Work out the finished part from the listing and answer in its coordinate system (mm). A direction names the side the tool comes from. Round coordinates to 2 decimals unless told otherwise and drop trailing zeros. Write each loop counter-clockwise with the first axis right and the second up, starting at its lowest first coordinate (ties: lowest second). Pieces come first, ordered by that corner, then holes.
1. Find section A-A (x = 0). Write down the section's boundary in (y, z).
2. Straight lines are drawn through the part: probe 1 along X at (y, z) = (2, 9); probe 2 along Z at (x, y) = (-33, 10); probe 3 along Y at (x, z) = (-16, 5). For each, find the intervals that lie inside material, in ascending order.
3. Flat-ended cylindrical pins translate along their axes: pin 1 Ø2 at (x, z) = (-28, -16) entering from -Y; pin 2 Ø4 at (x, z) = (-35, 8) entering from +Y; pin 3 Ø4.5 at (x, z) = (-37, 5.5) entering from +Y; pin 4 Ø2.5 at (x, z) = (-15.63, -6.22) entering from +Y. Find the tip coordinate at first contact, or state that the pin passes through.
4. Find section C-C (z = -2). Write down the section's boundary in (x, y).
5. Find section D-D (z = -24). Count the separate pieces of the cut face and the enclosed holes in it, and give its area (3 significant figures).
6. Find section B-B (y = 9.5). Write down the section's boundary in (x, z).
7. A tool of negligible diameter and unlimited length cuts with its end or side. For faces 5 (the face through (35, 5, -7)), 6 (the face through (-34, 3.75, 12)), 7 (the face through (-22.5, 10, -7)), 8 (the face through (-33, 9, 19)), from which of +Z, -Z, +X, -X, +Y, -Y can it reach the whole face along a straight path? Write none if from no direction.
8. Determine the mould class of faces 1 (the face through (-34, 3.75, -21)), 2 (the face through (-35, 5, -7)), 3 (the face through (-42.434, 2, -7)), 4 (the face through (28.36, 15.48, -33.1)) for opening direction X: pulls with the +X half, pulls with the -X half, needs draft (parallel to the pull), parting line crosses it, or undercut.
```python
from build123d import *

# Parameters (mm, degrees)
SKETCH1_W           = 50
SKETCH1_H           = 50
BOSS_EXTRUDE1_DEPTH = 30
SKETCH2_R           = 7
CUT_EXTRUDE1_DEPTH  = 30
SKETCH3_R           = 1.7
CUT_EXTRUDE2_DEPTH  = 42
SKETCH5_W           = 50
SKETCH5_H           = 15
BOSS_EXTRUDE2_DEPTH = 30
BOSS_EXTRUDE3_DEPTH = 65
SKETCH7_W           = 45
SKETCH7_H           = 42.253035939
CUT_EXTRUDE3_DEPTH  = 66
FILLET1_R           = 4
CUT_EXTRUDE4_DEPTH  = 53
SKETCH10_R          = 4
CUT_EXTRUDE5_DEPTH  = 1.25
SKETCH11_R          = 2.5
CUT_EXTRUDE6_DEPTH  = 36.25
CUT_EXTRUDE7_DEPTH  = 90.25
FILLET2_R           = 3
SKETCH13_W          = 3
SKETCH13_H          = 5
BOSS_EXTRUDE4_DEPTH = 65
FILLET3_R           = 3


with BuildPart() as part:
    # Sketch1 → Boss-Extrude1 (new body)
    with BuildSketch(Plane(origin=(0, 0, 0), x_dir=(1, 0, 0), z_dir=(0, 1, 0))):
        Rectangle(SKETCH1_W, SKETCH1_H)
    extrude(amount=BOSS_EXTRUDE1_DEPTH)

    # Sketch2 → Cut-Extrude1 (cut)
    with BuildSketch(Plane(origin=(0, 30, 0), x_dir=(1, 0, 0), z_dir=(0, 1, 0))):
        Circle(SKETCH2_R)
    extrude(amount=-CUT_EXTRUDE1_DEPTH, mode=Mode.SUBTRACT)

    # Sketch3 → Cut-Extrude2 (cut)
    with BuildSketch(Plane.XZ):
        with Locations((6.617670641, -20.610654448)):
            Circle(SKETCH3_R)
        with Locations((14.927003033, -7.763670553)):
            Circle(SKETCH3_R)
        with Locations((7.955854814, 5.855914334)):
            Circle(SKETCH3_R)
        with Locations((-7.324625797, 6.628515327)):
            Circle(SKETCH3_R)
        with Locations((-15.633958189, -6.218468568)):
            Circle(SKETCH3_R)
        with Locations((-8.66280997, -19.838053456)):
            Circle(SKETCH3_R)
    extrude(amount=-CUT_EXTRUDE2_DEPTH, mode=Mode.SUBTRACT)

    # Sketch5 → Boss-Extrude2 (add)
    with BuildSketch(Plane(origin=(0, 30, 0), x_dir=(1, 0, 0), z_dir=(0, 1, 0))):
        with Locations((0, 32.5)):
            Rectangle(SKETCH5_W, SKETCH5_H)
    extrude(amount=-BOSS_EXTRUDE2_DEPTH)

    # Sketch6 → Boss-Extrude3 (add)
    with BuildSketch(Plane.XY.offset(25)):
        Polygon((-25, 30), (-42.320508076, 0), (-25, 0), align=None)
    boss_extrude3 = extrude(amount=-BOSS_EXTRUDE3_DEPTH)

    # Mirror1: Boss-Extrude3 across plane
    add(boss_extrude3.mirror(Plane(origin=(0, 0, 0), x_dir=(0, 0, 1), z_dir=(1, 0, 0))))

    # Sketch7 → Cut-Extrude3 (cut)
    with BuildSketch(Plane.XY.offset(25)):
        with Locations((0, 3.87348203)):
            Rectangle(SKETCH7_W, SKETCH7_H)
    extrude(amount=-CUT_EXTRUDE3_DEPTH, mode=Mode.SUBTRACT)

    # Fillet1
    fillet1_edges = [part.edges().sort_by_distance(p)[0] for p in [
        (-22.5, 25, -7.5),
        (22.5, 25, -7.5),
    ]]
    fillet(fillet1_edges, radius=FILLET1_R)

    # Sketch9 → Cut-Extrude4 (cut)
    with BuildSketch(Plane.XY.offset(19)):
        Polygon((27.5, 25.669872981), (39.43375673, 5), (27.5, 5), align=None)
    cut_extrude4 = extrude(amount=-CUT_EXTRUDE4_DEPTH, mode=Mode.SUBTRACT)

    # Mirror2: Cut-Extrude4 across plane
    add(cut_extrude4.mirror(Plane(origin=(0, 0, 0), x_dir=(0, 0, 1), z_dir=(1, 0, 0))), mode=Mode.SUBTRACT)

    # Sketch10 → Cut-Extrude5 (cut)
    with BuildSketch(Plane(origin=(0, 5, 0), x_dir=(1, 0, 0), z_dir=(0, 1, 0))):
        with Locations((33.466878365, 24)):
            Circle(SKETCH10_R)
        with Locations((33.466878365, -9)):
            Circle(SKETCH10_R)
        with Locations((-33.466878365, -9)):
            Circle(SKETCH10_R)
        with Locations((-33.466878365, 24)):
            Circle(SKETCH10_R)
    extrude(amount=-CUT_EXTRUDE5_DEPTH, mode=Mode.SUBTRACT)

    # Sketch11 → Cut-Extrude6 (cut)
    with BuildSketch(Plane(origin=(0, 3.75, 0), x_dir=(1, 0, 0), z_dir=(0, 1, 0))):
        with Locations((33.466878365, 24)):
            Circle(SKETCH11_R)
        with Locations((33.466878365, -9)):
            Circle(SKETCH11_R)
        with Locations((-33.466878365, -9)):
            Circle(SKETCH11_R)
        with Locations((-33.466878365, 24)):
            Circle(SKETCH11_R)
    extrude(amount=-CUT_EXTRUDE6_DEPTH, mode=Mode.SUBTRACT)

    # Sketch12 → Cut-Extrude7 (cut)
    with BuildSketch(Plane.XY.offset(25)):
        Polygon((42.320508076, 0), (39.43375673, 5), (39.43375673, 0), align=None)
    cut_extrude7 = extrude(amount=-CUT_EXTRUDE7_DEPTH, mode=Mode.SUBTRACT)

    # Mirror3: Cut-Extrude7 across plane
    add(cut_extrude7.mirror(Plane(origin=(0, 0, 0), x_dir=(0, 0, 1), z_dir=(1, 0, 0))), mode=Mode.SUBTRACT)

    # Fillet2
    fillet2_edges = [part.edges().sort_by_distance(p)[0] for p in [
        (27.5, 15.334936491, 19),
        (27.5, 15.334936491, -34),
        (-27.5, 15.334936491, -34),
        (-27.5, 15.334936491, 19),
    ]]
    fillet(fillet2_edges, radius=FILLET2_R)

    # Sketch13 → Boss-Extrude4 (add)
    with BuildSketch(Plane.XY.offset(25)):
        with Locations((40.93375673, 2.5)):
            Rectangle(SKETCH13_W, SKETCH13_H)
    boss_extrude4 = extrude(amount=-BOSS_EXTRUDE4_DEPTH)

    # Mirror4: Boss-Extrude4 across plane
    add(boss_extrude4.mirror(Plane(origin=(0, 0, 0), x_dir=(0, 0, 1), z_dir=(1, 0, 0))))

    # Fillet3
    fillet3_edges = [part.edges().sort_by_distance(p)[0] for p in [
        (42.43375673, 2.5, -40),
        (42.43375673, 2.5, 25),
        (-42.43375673, 2.5, 25),
        (-42.43375673, 2.5, -40),
    ]]
    fillet(fillet3_edges, radius=FILLET3_R)


solid = part.part
```
Worked answers:
1. outline: (25, -40) - (30, -40) - (30, -7) - (25, -7) - close; (25, 7) - (30, 7) - (30, 25) - (25, 25) - close
2. probe 1: x = -42.43 to -35.97, -30.97 to -22.5, 22.5 to 30.97, 35.97 to 42.43
2. probe 2: z = -40 to -34, 19 to 25
2. probe 3: y = 25 to 30
3. pin 1: stops at y = 0
3. pin 2: stops at y = 3.75
3. pin 3: stops at y = 5
3. pin 4: passes through
4. outline: (-42.43, 0) - (-22.5, 0) - (-22.5, 21) arc R4 cw to (-18.5, 25) - (-6.71, 25) - (-6.71, 30) - (-25, 30) - (-27.5, 25.67) - (-27.5, 5) - (-42.43, 5) - close; (6.71, 25) - (18.5, 25) arc R4 cw to (22.5, 21) - (22.5, 0) - (42.43, 0) - (42.43, 5) - (27.5, 5) - (27.5, 25.67) - (25, 30) - (6.71, 30) - close
5. separate pieces: 3
5. enclosed holes: 0
5. area: 613 mm2
6. outline: (-36.84, -40) - (-22.5, -40) - (-22.5, 25) - (-36.84, 25) - (-36.84, 19) - (-30.5, 19) arc R3 cw to (-27.5, 16) - (-27.5, -31) arc R3 cw to (-30.5, -34) - (-36.84, -34) - close; (22.5, -40) - (36.84, -40) - (36.84, -34) - (30.5, -34) arc R3 cw to (27.5, -31) - (27.5, 16) arc R3 cw to (30.5, 19) - (36.84, 19) - (36.84, 25) - (22.5, 25) - close
7. face 5: +X, +Y
7. face 6: +Y
7. face 7: +Z, -Z, -Y
7. face 8: -X, +Y
8. face 1: undercut
8. face 2: needs draft
8. face 3: pulls with the -X half
8. face 4: pulls with the +X half
